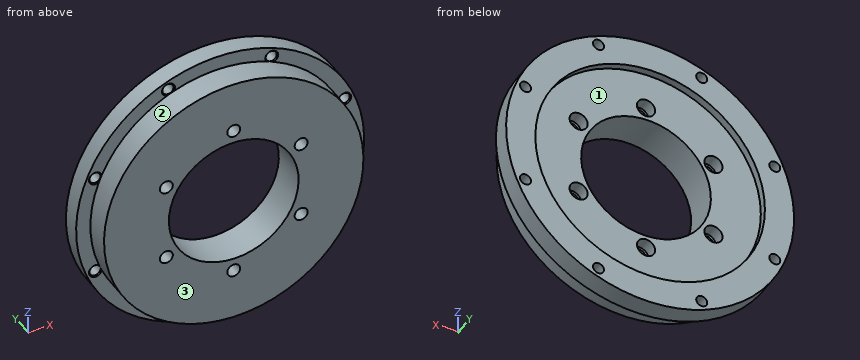
```python
from build123d import *

# Parameters (mm, degrees)
CUT_EXTRUDE1_REACH = 162.832
SKETCH3_R          = 5
SKETCH5_R          = 88.5
CUT_EXTRUDE3_DEPTH = 6
SKETCH4_R          = 7
CUT_EXTRUDE2_DEPTH = 10
CIRPATTERN1_COUNT  = 8


with BuildPart() as part:
    # Sketch1 → Revolve1 (revolve)
    with BuildSketch(Plane.XY, mode=Mode.PRIVATE) as revolve1_sk:
        Polygon((50, 0), (50, 35), (111, 35), (111, 20), (100, 20), (100, 0), align=None)
    revolve(revolve1_sk.sketch.rotate(Axis((0, 0, 0), (0, 1, 0)), 90), axis=Axis((0, 0, 0), (0, 1, 0)))

    # Sketch3 → Cut-Extrude1 (cut, up to next)
    with BuildSketch(Plane.XZ, mode=Mode.PRIVATE) as cut_extrude1_sk1:
        with Locations(Location((0, 60, 0), (0, 0, 270))):
            Circle(SKETCH3_R)
    cut_extrude1_tool1 = extrude(cut_extrude1_sk1.sketch, amount=-CUT_EXTRUDE1_REACH, mode=Mode.PRIVATE) & part.part
    # Sketch3 → Cut-Extrude1 (cut, up to next)
    with BuildSketch(Plane.XZ, mode=Mode.PRIVATE) as cut_extrude1_sk2:
        with Locations(Location((51.961524227, 30, 0), (0, 0, 270))):
            Circle(SKETCH3_R)
    cut_extrude1_tool2 = extrude(cut_extrude1_sk2.sketch, amount=-CUT_EXTRUDE1_REACH, mode=Mode.PRIVATE) & part.part
    # Sketch3 → Cut-Extrude1 (cut, up to next)
    with BuildSketch(Plane.XZ, mode=Mode.PRIVATE) as cut_extrude1_sk3:
        with Locations(Location((51.961524227, -30, 0), (0, 0, 270))):
            Circle(SKETCH3_R)
    cut_extrude1_tool3 = extrude(cut_extrude1_sk3.sketch, amount=-CUT_EXTRUDE1_REACH, mode=Mode.PRIVATE) & part.part
    # Sketch3 → Cut-Extrude1 (cut, up to next)
    with BuildSketch(Plane.XZ, mode=Mode.PRIVATE) as cut_extrude1_sk4:
        with Locations(Location((0, -60, 0), (0, 0, 270))):
            Circle(SKETCH3_R)
    cut_extrude1_tool4 = extrude(cut_extrude1_sk4.sketch, amount=-CUT_EXTRUDE1_REACH, mode=Mode.PRIVATE) & part.part
    # Sketch3 → Cut-Extrude1 (cut, up to next)
    with BuildSketch(Plane.XZ, mode=Mode.PRIVATE) as cut_extrude1_sk5:
        with Locations(Location((-51.961524227, -30, 0), (0, 0, 270))):
            Circle(SKETCH3_R)
    cut_extrude1_tool5 = extrude(cut_extrude1_sk5.sketch, amount=-CUT_EXTRUDE1_REACH, mode=Mode.PRIVATE) & part.part
    # Sketch3 → Cut-Extrude1 (cut, up to next)
    with BuildSketch(Plane.XZ, mode=Mode.PRIVATE) as cut_extrude1_sk6:
        with Locations(Location((-51.961524227, 30, 0), (0, 0, 270))):
            Circle(SKETCH3_R)
    cut_extrude1_tool6 = extrude(cut_extrude1_sk6.sketch, amount=-CUT_EXTRUDE1_REACH, mode=Mode.PRIVATE) & part.part
    add(cut_extrude1_tool1.solids().sort_by_distance((0, 0, 60))[0], mode=Mode.SUBTRACT)
    add(cut_extrude1_tool2.solids().sort_by_distance((51.961524, 0, 30))[0], mode=Mode.SUBTRACT)
    add(cut_extrude1_tool3.solids().sort_by_distance((51.961524, 0, -30))[0], mode=Mode.SUBTRACT)
    add(cut_extrude1_tool4.solids().sort_by_distance((0, 0, -60))[0], mode=Mode.SUBTRACT)
    add(cut_extrude1_tool5.solids().sort_by_distance((-51.961524, 0, -30))[0], mode=Mode.SUBTRACT)
    add(cut_extrude1_tool6.solids().sort_by_distance((-51.961524, 0, 30))[0], mode=Mode.SUBTRACT)

    # Sketch5 → Cut-Extrude3 (cut)
    with BuildSketch(Plane(origin=(0, 35, 0), x_dir=(1, 0, 0), z_dir=(0, 1, 0))):
        with Locations(Location((0, 0, 0), (0, 0, 270))):
            Circle(SKETCH5_R)
    extrude(amount=-CUT_EXTRUDE3_DEPTH, mode=Mode.SUBTRACT)

    # Sketch4 → Cut-Extrude2 (cut)
    with BuildSketch(Plane(origin=(0, 29, 0), x_dir=(1, 0, 0), z_dir=(0, 1, 0))):
        with Locations(Location((0, 60, 0), (0, 0, 270))):
            Circle(SKETCH4_R)
        with Locations(Location((51.961524227, 30, 0), (0, 0, 270))):
            Circle(SKETCH4_R)
        with Locations(Location((51.961524227, -30, 0), (0, 0, 270))):
            Circle(SKETCH4_R)
        with Locations(Location((0, -60, 0), (0, 0, 270))):
            Circle(SKETCH4_R)
        with Locations(Location((-51.961524227, -30, 0), (0, 0, 270))):
            Circle(SKETCH4_R)
        with Locations(Location((-51.961524227, 30, 0), (0, 0, 270))):
            Circle(SKETCH4_R)
    extrude(amount=-CUT_EXTRUDE2_DEPTH, mode=Mode.SUBTRACT)

    # Sketch8 → M10 Tapped Hole1 (revolve, cut)
    with BuildSketch(Plane(origin=(39.799076966, 20, 96.083471381), x_dir=(0, 0, -1), z_dir=(1, 0, 0))):
        Polygon((0, 0), (0, 27.053657631), (4.25, 24.5), (4.25, 0.775), (5.025, 0), align=None)
    m10_tapped_hole1 = revolve(axis=Axis((39.799076966, 13.65, 96.083471381), (0, 1, 0)), mode=Mode.SUBTRACT)

    # CirPattern1: M10 Tapped Hole1 ×8 about axis
    cirpattern1_axis = Axis((0, 0, 0), (0, 1, 0))
    for i in range(1, CIRPATTERN1_COUNT):
        add(m10_tapped_hole1.rotate(cirpattern1_axis, i * 360 / CIRPATTERN1_COUNT), mode=Mode.SUBTRACT)


solid = part.part
```
Geometry: final body of the model. Coordinates: model frame, mm. Face numbers are marked on the shaded views. Coordinates: 2 decimals unless noted, no trailing zeros. Write each loop counter-clockwise with the first axis right and the second up, starting at its lowest first coordinate (ties: lowest second). Pieces come first, ordered by that corner, then holes. Notation, with made-up numbers: M 73.5,-10.5 L 109.5,-10.5 A38 ccw 109.5,28.5 Z; hole C -8,69 d2. An arc over 180 degrees is marked long. Use CSV: the item, a comma, the result in double quotes. Start each with the question number.
1. Cut plane D-D on x = -66. Return the cut outline in (y, z).
2. Cut plane A-A on x = 0. Count the separate pieces of the cut face and the enclosed holes in it, plus the area to 3 significant figures.
3. Mould query, pull axis X, two halves, no side actions, for the marked faces 1, 2 and 3. Classes: pulls with the +X half, pulls with the -X half, needs draft (parallel to the pull), parting line crosses it, or undercut.
4. Ray query, probe 1 along Z at (x, y) = (96.5, 23.5); probe 2 along X at (y, z) = (22, 30); probe 3 along Y at (x, z) = (-74, 26). Return the intervals inside material, ascending.
5. Cut plane C-C on y = 5.5. Return the cut outline in (x, z).
6. First-contact query: P1, Ø11.5, axis at x = 51.96, z = 30, coming from the +Y side; P2, Ø3, axis at y = 8.5, z = 50.5, coming from the -X side; P3, Ø6, axis at y = 13.5, z = -74, coming from the -X side; P4, Ø7, axis at x = -96.08, z = -39.8, coming from the +Y side. Flat tips, straight axial feed; report the tip coordinate or a pass-through.
7. Cut plane B-B on z = 0. Return the cut outline in (x, y), plus the area to 3 significant figures.
Entries:
1,outline,"M 0,-75.13 L 20,-75.13 L 20,-89.25 L 35,-89.25 L 35,-58.96 L 29,-58.96 L 29,58.96 L 35,58.96 L 35,89.25 L 20,89.25 L 20,75.13 L 0,75.13 Z"
2,separate pieces,"4"
2,enclosed holes,"0"
2,area,"2,710 mm²"
3,face 1,"undercut"
3,face 2,"parting line crosses it"
3,face 3,"needs draft"
4,probe 1,"-54.85 to -44.03, -35.57 to 35.57, 44.03 to 54.85"
4,probe 2,"-106.87 to -58.96, -44.96 to -40, 40 to 44.96, 58.96 to 106.87"
4,probe 3,"0 to 29"
5,outline,"C 0,0 d200; hole C -51.96,-30 d10; hole C -51.96,30 d10; hole C 0,0 d100; hole C 0,-60 d10; hole C 0,60 d10; hole C 51.96,-30 d10; hole C 51.96,30 d10"
6,P1,"y = 19"
6,P2,"x = -87.17"
6,P3,"x = -70.42"
6,P4,"through"
7,outline,"M -111,20 L -100,20 L -100,0 L -50,0 L -50,29 L -88.5,29 L -88.5,35 L -111,35 Z; M 50,0 L 100,0 L 100,20 L 111,20 L 111,35 L 88.5,35 L 88.5,29 L 50,29 Z"
7,area,"3,370 mm²"
